Build history of the part. All positions in model axes, mm. Face numbers are marked on the shaded views. A direction names the side the tool comes from. Round coordinates to 2 decimals unless told otherwise and drop trailing zeros. Write each loop counter-clockwise with the first axis right and the second up, starting at its lowest first coordinate (ties: lowest second). Pieces come first, ordered by that corner, then holes. Notation, with made-up numbers: (66.5, 59.5) - (90.5, 59.5) arc R15 ccw to (90.5, 88.5) - close; hole circle Ø4 at (52.25, -13). An arc over 180 degrees is marked (long way). Answer as a JSON object with one key per item and string values. Group by question number.
Item 1: Slice it at B-B, the plane x = -32.5. List the corners of the cut face in (y, z), then the cut area to 3 significant figures.
Item 2: Two-plate mould, pull along X, no slides. Class the marked faces 1, 2, 3 and 4: +X half, -X half, draft (parallel to the pull), parting line (faces both ways), or undercut.
Item 3: Flat gauge pins, fed straight in: pin 1 (20.5 mm diameter, centred on x = 5.94, y = 80.95, fed in from +Z); pin 2 (8 mm diameter, centred on x = -28, y = 60, fed in from -Z). Where does each tip first touch, or does it go through?
Item 4: Probe line 1 (Y direction, x = -16, z = 4.5); line 2 (X direction, y = 4, z = 24); line 3 (Y direction, x = -6, z = 9.5). List the from-to ranges inside material, lowest first. Write a range as from..to.
Item 5: Which spindle directions (+Z, -Z, +X, -X, +Y, -Y) get a long thin tool onto all of the face, cutting with end or side? Do the marked faces 5 and 6. Say none if no direction does.
Item 6: Slice it at A-A, the plane y = -38. List the corners of the cut face in (x, z), then the cut area to 3 significant figures.
Item 7: Slice it at C-C, the plane z = 11. List the corners of the cut face in (x, y), then the cut area to 3 significant figures.
Item 8: Slice it at D-D, the plane x = -52.5. List the corners of the cut face in (y, z), then the cut area to 3 significant figures.
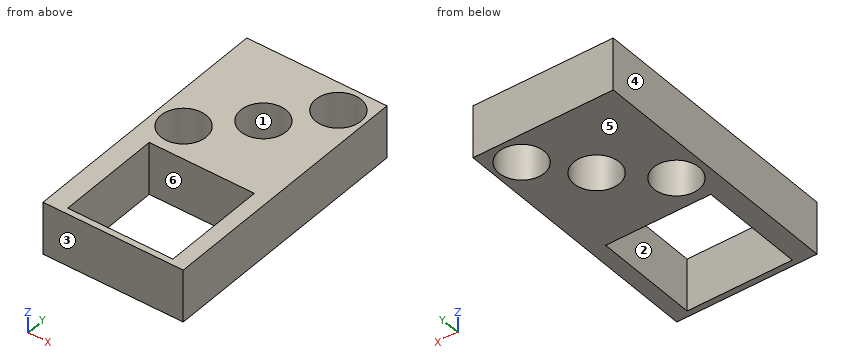
from build123d import *

# Parameters (mm, degrees)
SKETCH_W   = 80
SKETCH_H   = 150
SKETCH_R   = 12.93489
SKETCH_W_2 = 60
SKETCH_H_2 = 60
PAD_DEPTH  = 30


with BuildPart() as part:
    # Sketch → Pad (new body)
    with BuildSketch(Plane.XY):
        with Locations((-18.684139, 21.9223)):
            Rectangle(SKETCH_W, SKETCH_H)
        with Locations((-42.216557, 29.153965)):
            Circle(SKETCH_R, mode=Mode.SUBTRACT)
        with Locations((-16.072264, 54.191032)):
            Circle(SKETCH_R, mode=Mode.SUBTRACT)
        with Locations((5.941536, 80.952904)):
            Circle(SKETCH_R, mode=Mode.SUBTRACT)
        with Locations((-17.261113, -19.638437)):
            Rectangle(SKETCH_W_2, SKETCH_H_2, mode=Mode.SUBTRACT)
    extrude(amount=PAD_DEPTH)


solid = part.part
Geometry says:
{
 "1": {"outline": "(-53.08, 0) - (-49.64, 0) - (-49.64, 30) - (-53.08, 30) - close; (10.36, 0) - (20.62, 0) - (20.62, 30) - (10.36, 30) - close; (37.69, 0) - (96.92, 0) - (96.92, 30) - (37.69, 30) - close", "area": "2,190 mm^2"},
 "2": {"face 1": "undercut", "face 2": "undercut", "face 3": "draft", "face 4": "-X half"},
 "3": {"pin 1": "passes through", "pin 2": "stops at z = 0"},
 "4": {"line 1": "y = -53.08..-49.64, 10.36..41.26, 67.13..96.92", "line 2": "x = -58.68..-47.26, 12.74..21.32", "line 3": "y = -53.08..-49.64, 10.36..46.08, 62.31..75.98, 85.92..96.92"},
 "5": {"face 5": "-Z, +X, -X, +Y, -Y", "face 6": "+Z, -Z"},
 "6": {"outline": "(-58.68, 0) - (-47.26, 0) - (-47.26, 30) - (-58.68, 30) - close; (12.74, 0) - (21.32, 0) - (21.32, 30) - (12.74, 30) - close", "area": "600 mm^2"},
 "7": {"outline": "(-58.68, -53.08) - (21.32, -53.08) - (21.32, 96.92) - (-58.68, 96.92) - close; hole circle Ø25.87 at (-42.22, 29.15); hole (-47.26, -49.64) - (12.74, -49.64) - (12.74, 10.36) - (-47.26, 10.36) - close; hole circle Ø25.87 at (-16.07, 54.19); hole circle Ø25.87 at (5.94, 80.95)", "area": "6,820 mm^2"},
 "8": {"outline": "(-53.08, 0) - (21.31, 0) - (21.31, 30) - (-53.08, 30) - close; (37, 0) - (96.92, 0) - (96.92, 30) - (37, 30) - close", "area": "4,030 mm^2"}
}
